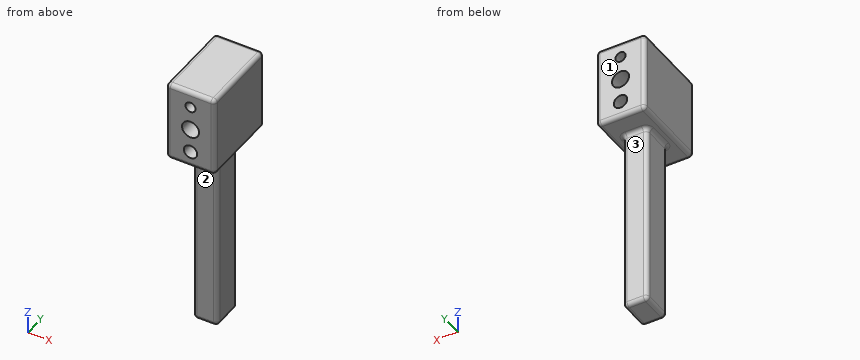
```python
from build123d import *

# Parameters (mm, degrees)
EXTRUDE_1_DEPTH     = 46
EXTRUDE_2_OUTLINE_W = 12
EXTRUDE_2_OUTLINE_H = 20
EXTRUDE_2_DEPTH     = 20
FILLET_1_R          = 1
FILLET_2_R          = 1
FILLET_3_R          = 1
FILLET_4_R          = 1
FILLET_5_R          = 1
HOLE_WIZARD_M5_1_D  = 4.2
HOLE_WIZARD_M4_1_D  = 3.3
HOLE_WIZARD_M3_1_D  = 2.5


# Read off the part's stored shape, not the designer's step: 凸台-拉伸2
with BuildPart() as part:
    # 草图1 → 凸台-拉伸1 (new body)
    with BuildSketch(Plane.XY):
        with BuildLine():
            Line((-2, -4), (2, -4))
            ThreePointArc((2, -4), (2.707106781, -3.707106781), (3, -3))
            Line((3, -3), (3, 3))
            ThreePointArc((3, 3), (2.707106781, 3.707106781), (2, 4))
            Line((2, 4), (-2, 4))
            ThreePointArc((-2, 4), (-2.707106781, 3.707106781), (-3, 3))
            Line((-3, 3), (-3, -3))
            ThreePointArc((-3, -3), (-2.707106781, -3.707106781), (-2, -4))
        make_face()
    extrude(amount=EXTRUDE_1_DEPTH)

    # 凸台-拉伸2 outline → 凸台-拉伸2 (add)
    with BuildSketch(Plane.XY.offset(46)):
        Rectangle(EXTRUDE_2_OUTLINE_W, EXTRUDE_2_OUTLINE_H)
    extrude(amount=EXTRUDE_2_DEPTH)

    # 圆角1
    fillet_1_edges = [part.edges().sort_by_distance(p)[0] for p in [
        (6, -10, 56),
        (6, 10, 56),
        (-6, 10, 56),
        (-6, -10, 56),
    ]]
    fillet(fillet_1_edges, radius=FILLET_1_R)

    # 圆角2
    fillet_2_edges = [part.edges().sort_by_distance(p)[0] for p in [
        (2.707106781, -3.707106781, 46),
        (3, 0, 46),
        (2.707106781, 3.707106781, 46),
        (0, 4, 46),
        (-2.707106781, 3.707106781, 46),
        (-3, 0, 46),
        (-2.707106781, -3.707106781, 46),
        (0, -4, 46),
    ]]
    fillet(fillet_2_edges, radius=FILLET_2_R)

    # 圆角3
    fillet_3_edges = [part.edges().sort_by_distance(p)[0] for p in [
        (0, -10, 66),
        (-6, 0, 66),
        (6, 0, 66),
        (0, 10, 66),
        (-5.707106781, 9.707106781, 66),
        (5.707106781, 9.707106781, 66),
        (5.707106781, -9.707106781, 66),
        (-5.707106781, -9.707106781, 66),
    ]]
    fillet(fillet_3_edges, radius=FILLET_3_R)

    # 圆角4
    fillet_4_edges = [part.edges().sort_by_distance(p)[0] for p in [
        (0, -10, 46),
        (6, 0, 46),
        (-6, 0, 46),
        (0, 10, 46),
        (-5.707106781, 9.707106781, 46),
        (5.707106781, 9.707106781, 46),
        (5.707106781, -9.707106781, 46),
        (-5.707106781, -9.707106781, 46),
    ]]
    fillet(fillet_4_edges, radius=FILLET_4_R)

    # 圆角5
    fillet_5_edges = [part.edges().sort_by_distance(p)[0] for p in [
        (3, 0, 0),
        (2.707106781, -3.707106781, 0),
        (0, -4, 0),
        (-2.707106781, -3.707106781, 0),
        (-3, 0, 0),
        (-2.707106781, 3.707106781, 0),
        (0, 4, 0),
        (2.707106781, 3.707106781, 0),
    ]]
    fillet(fillet_5_edges, radius=FILLET_5_R)

    # M5 螺纹孔1 (through all)
    with Locations(Plane(origin=(0, 10, 0), x_dir=(1, 0, 0), z_dir=(0, 1, 0))):
        with Locations((0, -56)):
            Hole(HOLE_WIZARD_M5_1_D / 2)

    # M4 螺纹孔1 (through all)
    with Locations(Plane(origin=(0, 10, 0), x_dir=(1, 0, 0), z_dir=(0, 1, 0))):
        with Locations((0, -50)):
            Hole(HOLE_WIZARD_M4_1_D / 2)

    # M3 螺纹孔1 (through all)
    with Locations(Plane(origin=(0, 10, 0), x_dir=(1, 0, 0), z_dir=(0, 1, 0))):
        with Locations((0, -62)):
            Hole(HOLE_WIZARD_M3_1_D / 2)


solid = part.part
```
Source: CAD feature listing. Evaluate the final solid. Frame: model axes, mm. Face numbers are marked on the shaded views. A direction names the side the tool comes from. Give positions to 0.01 mm unless a question says otherwise; leave off trailing zeros. Loops run counter-clockwise (first coordinate to the right, second up) from the corner with the lowest first, then second, coordinate; pieces in that order, holes last. Notation, with made-up numbers: (39, 50) -> (81, 50) arc R23 cw to (81, 85) -> close; hole circle Ø11 at (-16, 44). An arc over 180 degrees is marked (long way). Put each result on its own line as item: value. Start each with the question number.
1) Material intervals for probe 1 along Z at (x, y) = (0, 0.25); probe 2 along Z at (x, y) = (0, -5.5); probe 3 along X at (y, z) = (-3.75, 56), sorted ascending.
2) Reachability of the marked faces 1, 2 and 3 from +Z, -Z, +X, -X, +Y, -Y: full face, straight path, thin tool, end or side. Return the list, or none.
3) Cut plane B-B (x = 0). Return loops of the section in (y, z).
4) Cut plane D-D (z = 9). Return loops of the section in (x, y).
5) Cut plane A-A (z = 62). Return loops of the section in (x, y).
6) Cut plane C-C (y = -8). Return loops of the section in (x, z), then the cut area to 3 significant figures.
7) Contact query for flat-ended pins moving along their axis: P1, Ø2, axis at x = -0.5, z = 17.5, coming from the -Y side; P2, Ø3, axis at y = -0.5, z = 41, coming from the +X side; P3, Ø3, axis at y = 0, z = 20.5, coming from the -X side; P4, Ø5, axis at x = 0, z = 56, coming from the -Y side. Output: stop coordinate, or through.
Results are:
1. probe 1: z = 0 to 48.35, 51.65 to 53.9, 58.1 to 60.75, 63.25 to 66
1. probe 2: z = 46 to 48.35, 51.65 to 53.9, 58.1 to 60.75, 63.25 to 66
1. probe 3: x = -6 to -2.1, 2.1 to 6
2. face 1: +Z, -Z, +X, -X, +Y
2. face 2: -Z, +X, -X, -Y
2. face 3: -Z, +X, -X, +Y
3. outline: (-10, 47) arc R1 ccw to (-9, 46) -> (-5, 46) arc R1 cw to (-4, 45) -> (-4, 1) arc R1 ccw to (-3, 0) -> (3, 0) arc R1 ccw to (4, 1) -> (4, 45) arc R1 cw to (5, 46) -> (9, 46) arc R1 ccw to (10, 47) -> (10, 48.35) -> (-10, 48.35) -> close; (-10, 51.65) -> (10, 51.65) -> (10, 53.9) -> (-10, 53.9) -> close; (-10, 58.1) -> (10, 58.1) -> (10, 60.75) -> (-10, 60.75) -> close; (-10, 63.25) -> (10, 63.25) -> (10, 65) arc R1 ccw to (9, 66) -> (-9, 66) arc R1 ccw to (-10, 65) -> close
4. outline: (-3, -3) arc R1 ccw to (-2, -4) -> (2, -4) arc R1 ccw to (3, -3) -> (3, 3) arc R1 ccw to (2, 4) -> (-2, 4) arc R1 ccw to (-3, 3) -> close
5. outline: (-6, -9) arc R1 ccw to (-5, -10) -> (-1.25, -10) -> (-1.25, 10) -> (-5, 10) arc R1 ccw to (-6, 9) -> close; (1.25, -10) -> (5, -10) arc R1 ccw to (6, -9) -> (6, 9) arc R1 ccw to (5, 10) -> (1.25, 10) -> close
6. outline: (-6, 47) arc R1 ccw to (-5, 46) -> (5, 46) arc R1 ccw to (6, 47) -> (6, 65) arc R1 ccw to (5, 66) -> (-5, 66) arc R1 ccw to (-6, 65) -> close; hole circle Ø4.2 at (0, 56); hole circle Ø3.3 at (0, 50); hole circle Ø2.5 at (0, 62)
6. area: 212 mm2
7. P1: stops at y = -4
7. P2: stops at x = 3
7. P3: stops at x = -3
7. P4: stops at y = -10
